The model under review builds one solid part; all positions refer to its coordinate system, in mm. A direction names the side the tool comes from. Give positions to 0.01 mm unless a question says otherwise; leave off trailing zeros. Order: outer loops, then holes, each group sorted by start corner. A loop starts at its lowest first (then second) coordinate and runs counter-clockwise, first axis right, second up.
```python
from build123d import *

# Parameters (mm, degrees)
F0_W     = 5.0387987867
F0_H     = 19.8329761624
F0_R     = 2.8154783611
F0_R_2   = 2.8155
F0_W_2   = 4.9696583821
F1_DEPTH = 7
F2_W     = 17.0454550534
F2_H     = 9.2045464553
F3_DEPTH = 25


with BuildPart() as f1:
    # F0 (on Top) → F1 (new body)
    with BuildSketch(Plane.XY):
        with BuildLine():
            ThreePointArc((4.9696583821, 15.8411743726), (0, 14.8370421052), (-4.9696583821, 15.8411743726))
            Line((-4.9696583821, 15.8411743726), (-4.9696583821, 12.3679572716))
            Line((-4.9696583821, 12.3679572716), (-4.9696583821, -13.2841039449))
            Line((-4.9696583821, -13.2841039449), (-4.9696583821, -19.3917378783))
            Line((-4.9696583821, -19.3917378783), (0, -19.3917378783))
            Line((0, -19.3917378783), (5.0387987867, -19.3917378783))
            Line((5.0387987867, -19.3917378783), (5.0387987867, -11.8726156652))
            Line((5.0387987867, -11.8726156652), (5.0387987867, 12.3679572716))
            Line((5.0387987867, 12.3679572716), (5.0387987867, 15.8411743726))
            Line((5.0387987867, 15.8411743726), (4.9696583821, 15.8411743726))
        make_face()
        with BuildLine():
            Line((13.2841020823, 12.3679572716), (5.0387987867, 12.3679572716))
            Line((5.0387987867, 12.3679572716), (5.0387987867, -11.8726156652))
            ThreePointArc((5.0387987867, -11.8726156652), (10.8629911852, -15.3395790039), (13.2841020823, -9.0087596327))
            Line((13.2841020823, -9.0087596327), (13.2841020823, 12.3679572716))
        make_face()
        with BuildLine():
            Line((-4.9696583821, -13.2841039449), (-4.9696583821, 12.3679572716))
            Line((-4.9696583821, 12.3679572716), (-12.0625765994, 12.3679572716))
            Line((-12.0625765994, 12.3679572716), (-12.0625765994, -10.2302869782))
            ThreePointArc((-12.0625765994, -10.2302869782), (-10.0908850734, -15.4148140408), (-4.9696583821, -13.2841039449))
        make_face()
        with BuildLine():
            Line((5.0387987867, -39.2247140408), (0, -39.2247140408))
            Line((0, -39.2247140408), (0, -44.0338738263))
            add(Edge.make_bspline(
                [(5.0387987867, -39.2247140408), (7.2849400651, -41.0469321938), (12.2823824367, -45.1011875053), (4.3610338087, -44.4128386617), (0, -44.0338738263)],
                knots=[0, 0, 0, 0, 0.4494581651, 1, 1, 1, 1], degree=3))
        make_face()
        with Locations((2.5193993933, -29.3082259595)):
            Rectangle(F0_W, F0_H)
        with BuildLine():
            ThreePointArc((4.9696583821, 15.8411743726), (10.6642305698, 20.5579047033), (12.8, 27.6370421052))
            ThreePointArc((12.8, 27.6370421052), (-7.0791374019, 38.301272675), (-4.9696583821, 15.8411743726))
            ThreePointArc((-4.9696583821, 15.8411743726), (0, 14.8370421052), (4.9696583821, 15.8411743726))
        make_face()
        with Locations((-5.0387978554, 32.2177670896)):
            Circle(F0_R, mode=Mode.SUBTRACT)
        with Locations((4.6588750556, 32.61211887)):
            Circle(F0_R_2, mode=Mode.SUBTRACT)
        with BuildLine():
            Line((0, -39.2247140408), (-4.9696583821, -39.2247140408))
            add(Edge.make_bspline(
                [(-4.9696583821, -39.2247140408), (-7.8188484205, -41.0482913635), (-14.1279975934, -45.086358745), (-5.0037621436, -44.4066360778), (0, -44.0338738263)],
                knots=[0, 0, 0, 0, 0.4515965561, 1, 1, 1, 1], degree=3))
            Line((0, -44.0338738263), (0, -39.2247140408))
        make_face()
        with Locations((-2.484829191, -29.3082259595)):
            Rectangle(F0_W_2, F0_H)
    extrude(amount=F1_DEPTH)

    # F2 (on Top) → F3 (join)
    with BuildSketch(Plane.XY):
        with Locations((9.313e-07, -11.9318186771)):
            Rectangle(F2_W, F2_H)
    extrude(amount=F3_DEPTH)


solid = f1.part
```
Item 1: For faces 1 (the flat face through (-12.063, 1, 3)), 2 (the flat face through (13.284, 2, 3)), 3 (the flat face through (9, 12.368, 3)), list the 3-axis set-ups (+Z, -Z, +X, -X, +Y, -Y) from which the entire face can be reached by the end or side of a thin tool; tool diameter is ignored.
Values found:
face 1: +Z, -Z, -X
face 2: +Z, -Z, +X, +Y
face 3: +Z, -Z, +X
Item 2: For line 1 (Y direction, x = -7, z = 2); line 2 (Y direction, x = -9, z = 1.5); line 3 (Y direction, x = -6.5, z = 20), list the stretches that pass through material, from the lowest coordinate up.
Values found:
line 1: y = -44.42 to -40.54, -16.53 to 12.37, 16.92 to 30.2, 34.24 to 38.35
line 2: y = -44.32 to -41.96, -15.7 to 12.37, 18.54 to 36.74
line 3: y = -16.53 to -7.33
Item 3: Draft analysis for pull direction Y (two halves, no side actions). For faces 4 (the flat face through (0, -7.33, 16)), 5 (the flat face through (5.039, 14, 3)), 6 (the flat face through (-1, -31, 7)), state which applies: released by +Y, released by -Y, zero draft, split by the parting line, or undercut.
Values found:
face 4: released by +Y
face 5: undercut
face 6: zero draft
Item 4: Take a section at A-A (y = 6). Give the boundary of the cut face in (x, z), and give its area (3 significant figures).
Values found:
outline: (-12.06, 0) - (13.28, 0) - (13.28, 7) - (-12.06, 7) - close
area: 177 mm2
Item 5: Take a section at B-B (z = 20). Give the boundary of the cut face in (x, y), and give its area (3 significant figures).
Values found:
outline: (-8.52, -16.53) - (8.52, -16.53) - (8.52, -7.33) - (-8.52, -7.33) - close
area: 157 mm2
Item 6: Take a section at C-C (z = 3.25). Give the number of separate pieces and of enclosed holes in the cut face, and give its area (3 significant figures).
Values found:
separate pieces: 1
enclosed holes: 2
area: 1,520 mm2
Item 7: Clearance check with flat-ended pins moving along their axes: pin 1 Ø5.5 at (y, z) = (-24, 2.5) entering from -X; pin 2 Ø2 at (y, z) = (-26.5, 4) entering from +X; pin 3 Ø3 at (x, z) = (-1.5, 6.5) entering from -Y; pin 4 Ø3 at (y, z) = (-18.5, 11) entering from -X. State where each tip first meets the part, or that it passes through.
Values found:
pin 1: stops at x = -4.97
pin 2: stops at x = 5.04
pin 3: stops at y = -44.25
pin 4: passes through
